Geometry check sheet. Reference: the model listing, model coordinates, mm. A direction names the side the tool comes from. Coordinates: 2 decimals unless noted, no trailing zeros. Order: outer loops, then holes, each group sorted by start corner. A loop starts at its lowest first (then second) coordinate and runs counter-clockwise, first axis right, second up. Notation, with made-up numbers: (18, 68) - (28, 68) arc R10 cw to (28, 76) - close; hole circle Ø11 at (-10.75, 86). An arc over 180 degrees is marked (long way). One line per item, written item: value. Start each with the question number.
```python
from build123d import *

# Parameters (mm, degrees)
RESSALTO_EXTRUS_O1_DEPTH                             = 4
FURO_DE_DI_METRO_6_0_6_1_D                           = 6
FURO_DE_DI_METRO_6_0_6_1_DEPTH                       = 2
FURO_DE_DI_METRO_6_0_6_1_TIP                         = 1.802581857
ESBO_O4_R                                            = 1.2
CORTE_EXTRUS_O1_DEPTH                                = 30.283417381
ESCAREADO_PARA_PARAFUSO_COM_CABE_A_ESCAR_D           = 3.4
ESCAREADO_PARA_PARAFUSO_COM_CABE_A_ESCAR_CSINK_D     = 6.3
ESCAREADO_PARA_PARAFUSO_COM_CABE_A_ESCAR_CSINK_ANGLE = 90


with BuildPart() as part:
    # Esboço1 → Ressalto-extrusão1 (new body)
    with BuildSketch(Plane(origin=(0, 0, 0), x_dir=(0, 0, -1), z_dir=(1, 0, 0))):
        with BuildLine():
            Line((0, 0), (0, 3.091839499))
            ThreePointArc((0, 3.091839499), (2.870368785, 6.92901728), (7.361966659, 5.259137398))
            Line((7.361966659, 5.259137398), (12.225984495, -9.134144996))
            Line((12.225984495, -9.134144996), (22, -18.908160501))
            Line((22, -18.908160501), (11, -18.908160501))
            Line((11, -18.908160501), (8, -15.908160501))
            Line((8, -15.908160501), (8, -8.399335203))
            Line((8, -8.399335203), (0, 0))
        make_face()
    extrude(amount=RESSALTO_EXTRUS_O1_DEPTH)

    # Furo de diâmetro Ø6.0 (6)1
    with Locations(Plane.ZY):
        with Locations((-4, 3.091839499)):
            Hole(FURO_DE_DI_METRO_6_0_6_1_D / 2, depth=FURO_DE_DI_METRO_6_0_6_1_DEPTH)
            with Locations((0, 0, -(FURO_DE_DI_METRO_6_0_6_1_DEPTH + FURO_DE_DI_METRO_6_0_6_1_TIP / 2))):  # 118° drill point
                Cone(0, FURO_DE_DI_METRO_6_0_6_1_D / 2, FURO_DE_DI_METRO_6_0_6_1_TIP, mode=Mode.SUBTRACT)

    # Esboço4 → Corte-extrusão1 (cut, through all)
    with BuildSketch(Plane(origin=(4, 0, 0), x_dir=(0, 0, -1), z_dir=(1, 0, 0))):
        with Locations((4, 3.091839499)):
            Circle(ESBO_O4_R)
    extrude(amount=-CORTE_EXTRUS_O1_DEPTH, mode=Mode.SUBTRACT)

    # Escareado para parafuso com cabeça escareada chata de M31 (through all)
    with Locations(Plane(origin=(4, 0, 0), x_dir=(0, 0, -1), z_dir=(1, 0, 0))):
        with Locations((13, -15.408160501)):
            CounterSinkHole(ESCAREADO_PARA_PARAFUSO_COM_CABE_A_ESCAR_D / 2, ESCAREADO_PARA_PARAFUSO_COM_CABE_A_ESCAR_CSINK_D / 2, counter_sink_angle=ESCAREADO_PARA_PARAFUSO_COM_CABE_A_ESCAR_CSINK_ANGLE)


solid = part.part
```
Q1. Set-up check for faces 1 (the flat face through (1.97, -13.95, -17.04)), 2 (the flat face through (2, -12, -8)), 3 (the cylindrical face through (1.01, 5.12, -1.79)): record each of +Z, -Z, +X, -X, +Y, -Y from which the full face is reachable in a straight line by a thin tool's end or side.
Q2. Cross-section at C-C, the plane z = -4. Enter the section's corners in (x, y), and give its area (3 significant figures).
Q3. Material ranges on probe 1 along Y at (x, z) = (3, -4.75); probe 2 along Y at (x, z) = (0.9, -4); probe 3 along Z at (x, y) = (0.55, -16.5), recorded low to high.
Q4. Release check for a two-part mould opening along Z. For faces 4 (the flat face through (2, 2, 0)), 5 (the cylindrical face through (3.55, 4.28, -3.84)), 6 (the cylindrical face through (1.972, 6.908, -2.802)) record: released by +Z, released by -Z, zero draft, split by the parting line, or undercut.
Q5. Gauge pin test, flat ends, axial feed: P1, Ø1.5, axis at x = 1.5, z = -3, coming from the -Y side; P2, Ø5, axis at y = 3.09, z = -4, coming from the -X side; P3, Ø1.2, axis at x = 1, y = -11, coming from the +Z side; P4, Ø1.4, axis at y = 3.09, z = -4, coming from the -X side. Record the tip position at first contact, or that the pin passes through.
Q6. Cross-section at A-A, the plane z = -13. Enter the section's corners in (x, y), and give its area (3 significant figures).
Q7. Cross-section at D-D, the plane z = -17.5. Enter the section's corners in (x, y).
Q8. Cross-section at B-B, the plane x = 1.6. Enter the section's corners in (y, z), and give its area (3 significant figures).
Check result:
1. face 1: -Z, +X, -X, +Y
1. face 2: +Z, +X, -X, -Y
1. face 3: -X
2. outline: (0, -4.2) - (4, -4.2) - (4, 1.89) - (3.08, 1.89) - (2, 0.09) - (0, 0.09) - close; (0, 6.09) - (2, 6.09) - (3.08, 4.29) - (4, 4.29) - (4, 7.09) - (0, 7.09) - close
2. area: 26.4 mm2
3. probe 1: y = -4.99 to 1.99, 4.2 to 7.02
3. probe 2: y = -4.2 to 0.09, 6.09 to 7.09
3. probe 3: z = -19.59 to -14.3, -11.7 to -8.59
4. face 4: released by +Z
4. face 5: undercut
4. face 6: split by the parting line
5. P1: stops at y = -3.94
5. P2: stops at x = 2.3
5. P3: stops at z = -8
5. P4: passes through
6. outline: (0, -18.91) - (4, -18.91) - (4, -18.56) - (2.55, -17.11) - (0, -17.11) - close; (0, -13.71) - (2.55, -13.71) - (4, -12.26) - (4, -9.91) - (0, -9.91) - close
6. area: 20.3 mm2
7. outline: (0, -18.91) - (4, -18.91) - (4, -14.41) - (0, -14.41) - close
8. outline: (-18.91, -22) - (-9.13, -12.23) - (5.26, -7.36) arc R4 ccw to (3.09, 0) - (0, 0) - (-8.4, -8) - (-15.91, -8) - (-18.91, -11) - close; hole circle Ø3.4 at (-15.41, -13); hole circle Ø6 at (3.09, -4)
8. area: 157 mm2
